Part model, mm, in its own coordinate system. Round coordinates to 2 decimals unless told otherwise and drop trailing zeros. Write each loop counter-clockwise with the first axis right and the second up, starting at its lowest first coordinate (ties: lowest second). Pieces come first, ordered by that corner, then holes. Notation, with made-up numbers: M 59,3.5 L 115,3.5 A21 ccw 115,10.5 Z; hole C 82.5,-22.5 d1. An arc over 180 degrees is marked long. Answer as a JSON object with one key per item and string values. Group by question number.
1. Band-saw the part on A-A, the plane y = -7. Write the cut outline in (x, z), plus the area to 3 significant figures.
2. Drill centre lines: line 1 (Y direction, x = -2.25, z = 0) (3 decimals); line 2 (X direction, y = -7, z = 0); line 3 (Y direction, x = 10.75, z = 0). Where is each one in solid material? Low to high. Write a range as from..to.
3. Band-saw the part on B-B, the plane z = 0. Write the cut outline in (x, y) (3 decimals), plus the area to 3 significant figures.
4. Band-saw the part on C-C, the plane x = -2. Write the cut outline in (y, z) (3 decimals), plus the area to 3 significant figures.
5. Drop a flat-ended pin along its axis: pin 1 (10 mm diameter, centred on x = 6, y = 2.5, fed in from +Z). Give the stop position or say it passes through.
Autodesk Inventor part; units mm, degrees
ref_plane "YZ Plane" through (0, 0, 0) normal (1, 0, 0) x (0, 1, 0)
ref_plane "XZ Plane" through (0, 0, 0) normal (0, 1, 0) x (-1, 0, 0)
ref_plane "XY Plane" through (0, 0, 0) normal (0, 0, 1) x (1, 0, 0)
sketch "Sketch1" plane through (0, 0, 0) normal (0, 0, 1) x (1, 0, 0)
  line L0 (-6.5, 7.175) -> (6.5, 7.175)
  line L1 (6.5, 7.175) -> (6.5, -7.175)
  line L2 (6.5, -7.175) -> (-6.5, -7.175)
  line L3 (-6.5, -7.175) -> (-6.5, 7.175)
  line L4 (8.8, 12.475) -> (-8.8, 12.475)
  line L5 (-11.8, 9.475) -> (-11.8, -9.475)
  line L6 (-8.8, -12.475) -> (8.8, -12.475)
  line L7 (11.8, -9.475) -> (11.8, 9.475)
  arc A0 (-8.8, 12.475) -> (-11.8, 9.475) centre (-8.8, 9.475) ccw
  arc A1 (11.8, 9.475) -> (8.8, 12.475) centre (8.8, 9.475) ccw
  arc A2 (8.8, -12.475) -> (11.8, -9.475) centre (8.8, -9.475) ccw
  arc A3 (-11.8, -9.475) -> (-8.8, -12.475) centre (-8.8, -9.475) ccw
  line L8 (7, 7.675) -> (-7, 7.675)
  line L9 (-7, 7.675) -> (-7, -7.675)
  line L10 (-7, -7.675) -> (7, -7.675)
  line L11 (7, -7.675) -> (7, 7.675)
  point P0 (0, 0)
  dimension "d0" = 13
  dimension "d1" = 14.35
  dimension "d3" = 3
  dimension "d4" = 7.175
  dimension "d5" = 6.5
  dimension "d11" = 0.5
  dimension "d12" = 24.95
  dimension "d13" = 23.6
sketch "Sketch2" plane through (0, 0, 0) normal (0, 1, 0) x (-1, 0, 0)
  circle A0 centre (-11.8, 0) radius 0.15
  point P0 (0, 0)
  dimension "d6" = 0.3
sweep "Sweep1" add profiles "Sketch2" path "Sketch1" path curves L5 A0 L4 A1 L7 A2 L6 A3
extrude "Extrusion1" add sketch "Sketch1" along normal mid plane 0.3 contours A1 L7 A2 L6 A3 L5 A0 L4
properties part number "COTS_GENERIC_Transformer_Electromagnet_Coil_Layer" material "Copper"
Worked answers:
{
 "1": {"outline": "M -11.8,-0.15 L -7,-0.15 L -7,0.15 L -11.8,0.15 A0.15 ccw Z; M 7,-0.15 L 11.8,-0.15 A0.15 ccw 11.8,0.15 L 7,0.15 Z", "area": "2.95 mm^2"},
 "2": {"line 1": "y = -12.625..-7.675, 7.675..12.625", "line 2": "x = -11.95..-7, 7..11.95", "line 3": "y = -11.95..11.95"},
 "3": {"outline": "M -11.95,-9.475 A3.15 ccw -8.8,-12.625 L 8.8,-12.625 A3.15 ccw 11.95,-9.475 L 11.95,9.475 A3.15 ccw 8.8,12.625 L -8.8,12.625 A3.15 ccw -11.95,9.475 Z; hole M -7,-7.675 L 7,-7.675 L 7,7.675 L -7,7.675 Z", "area": "380 mm^2"},
 "4": {"outline": "M -12.475,-0.15 L -7.675,-0.15 L -7.675,0.15 L -12.475,0.15 A0.15 ccw Z; M 7.675,-0.15 L 12.475,-0.15 A0.15 ccw 12.475,0.15 L 7.675,0.15 Z", "area": "2.95 mm^2"},
 "5": {"pin 1": "stops at z = 0.15"}
}
